The model under review builds one solid part; all positions refer to its coordinate system, in mm. A direction names the side the tool comes from. Coordinates: 2 decimals unless noted, no trailing zeros. Order: outer loops, then holes, each group sorted by start corner. A loop starts at its lowest first (then second) coordinate and runs counter-clockwise, first axis right, second up. Notation, with made-up numbers: (29, 53) - (71, 53) arc R21 cw to (71, 76) - close; hole circle Ø5 at (48, -14). An arc over 180 degrees is marked (long way). Answer in a Markdown table with one row per item.
```python
from build123d import *

# Parameters (mm, degrees)
BOSS_EXTRUDE1_DEPTH = 50
SHELL1_T            = -5
SKETCH5_W           = 10
SKETCH5_H           = 20
CUT_EXTRUDE1_DEPTH  = 5


with BuildPart() as part:
    # Sketch1 → Boss-Extrude1 (new body)
    with BuildSketch(Plane(origin=(0, 0, 0), x_dir=(1, 0, 0), z_dir=(0, 1, 0))):
        Polygon((-50, 80), (-80, 50), (-80, -50), (-50, -80), (50, -80), (80, -50), (80, 50), (50, 80), align=None)
    extrude(amount=BOSS_EXTRUDE1_DEPTH)

    # Shell1
    shell1_openings = [part.faces().sort_by_distance(p)[0] for p in [
        (0, 50, 0),
    ]]
    offset(amount=SHELL1_T, openings=shell1_openings, kind=Kind.INTERSECTION)

    # Sketch5 → Cut-Extrude1 (cut)
    with BuildSketch(Plane(origin=(0, 5, 0), x_dir=(1, 0, 0), z_dir=(0, 1, 0))):
        with Locations((-70, 0)):
            Rectangle(SKETCH5_W, SKETCH5_H)
    extrude(amount=-CUT_EXTRUDE1_DEPTH, mode=Mode.SUBTRACT)


solid = part.part
```
Item 1: Mouldability with a two-part tool opening along X and no side actions: class faces 4 (the face through (80, 25, 1)), 5 (the face through (-65, 25, -65)), 6 (the face through (-75, 25, 1)), 7 (the face through (-70, 3, 10)) as +X half, -X half, draft (parallel to the pull), parting line (faces both ways), or undercut.
Check values:
| item | result |
|---|---|
| face 4 | +X half |
| face 5 | -X half |
| face 6 | undercut |
| face 7 | undercut |
Item 2: Clearance check with flat-ended pins moving along their axes: pin 1 Ø5.5 at (x, y) = (-70.5, 3.5) entering from -Z; pin 2 Ø1 at (x, z) = (29, -20) entering from +Y; pin 3 Ø2.5 at (x, y) = (-69.5, 1.5) entering from +Z. State where each tip first meets the part, or that it passes through.
Check values:
| item | result |
|---|---|
| pin 1 | z = -62.25 |
| pin 2 | y = 5 |
| pin 3 | z = 61.75 |
Item 3: We need section A-A, the plane x = -67. Write out the cut boundary in (y, z).
Check values:
| item | result |
|---|---|
| outline | (0, -63) - (50, -63) - (50, -55.93) - (5, -55.93) - (5, -10) - (0, -10) - close; (0, 10) - (5, 10) - (5, 55.93) - (50, 55.93) - (50, 63) - (0, 63) - close |
Item 4: Tool access review of faces 1 (the face through (-1, 0, -1)), 2 (the face through (-70, 3, -10)), 3 (the face through (-1, 5, -1)): name each direction out of +Z, -Z, +X, -X, +Y, -Y from which nothing blocks a thin tool from reaching the whole face with its end or side.
Check values:
| item | result |
|---|---|
| face 1 | +Z, -Z, +X, -X, -Y |
| face 2 | +Y, -Y |
| face 3 | +Y |
Item 5: To check wall thickness, follow line 1 (X direction, y = 23, z = 45.5); line 2 (Y direction, x = 60, z = -38). State the ranges of each line that lie inside material, in increasing order. Write a range as from..to.
Check values:
| item | result |
|---|---|
| line 1 | -80..-75, 75..80 |
| line 2 | 0..5 |
Item 6: We need section B-B, the plane y = 21. Write out the cut boundary in (x, z), then the cut area to 3 significant figures.
Check values:
| item | result |
|---|---|
| outline | (-80, -50) - (-50, -80) - (50, -80) - (80, -50) - (80, 50) - (50, 80) - (-50, 80) - (-80, 50) - close; hole (-75, -47.93) - (-47.93, -75) - (47.93, -75) - (75, -47.93) - (75, 47.93) - (47.93, 75) - (-47.93, 75) - (-75, 47.93) - close |
| area | 2,770 mm^2 |
Item 7: We need section D-D, the plane x = -36. Write out the cut boundary in (y, z).
Check values:
| item | result |
|---|---|
| outline | (0, -80) - (50, -80) - (50, -75) - (5, -75) - (5, 75) - (50, 75) - (50, 80) - (0, 80) - close |
Item 8: We need section C-C, the plane z = 16. Write out the cut boundary in (x, y).
Check values:
| item | result |
|---|---|
| outline | (-80, 0) - (80, 0) - (80, 50) - (75, 50) - (75, 5) - (-75, 5) - (-75, 50) - (-80, 50) - close |
